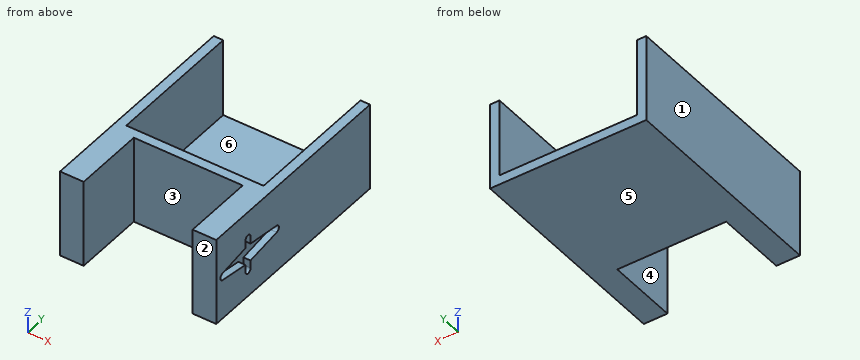
```python
from build123d import *

# Parameters (mm, degrees)
SKETCH_W        = 66
SKETCH_H        = 66
PAD_DEPTH       = 37
SKETCH001_W     = 58
SKETCH001_H     = 58
POCKET_DEPTH    = 33
SKETCH002_W     = 10
SKETCH002_H     = 37
PAD001_DEPTH    = 30
SKETCH003_W     = 66
SKETCH003_H     = 37
POCKET001_DEPTH = 4
POCKET002_DEPTH = 3


with BuildPart() as part:
    # Sketch → Pad (new body)
    with BuildSketch(Plane.XY):
        Rectangle(SKETCH_W, SKETCH_H)
    extrude(amount=PAD_DEPTH)

    # Sketch001 → Pocket (cut)
    with BuildSketch(Plane.XY.offset(37)):
        Rectangle(SKETCH001_W, SKETCH001_H)
    extrude(amount=-POCKET_DEPTH, mode=Mode.SUBTRACT)

    # Sketch002 → Pad001 (new body)
    with BuildSketch(Plane.XZ.offset(33)):
        with Locations((-28, 18.5)):
            Rectangle(SKETCH002_W, SKETCH002_H)
        with Locations((28, 18.5)):
            Rectangle(SKETCH002_W, SKETCH002_H)
    extrude(amount=PAD001_DEPTH)

    # Sketch003 → Pocket001 (cut)
    with BuildSketch(Plane(origin=(0, 33, 0), x_dir=(-1, 0, 0), z_dir=(0, 1, 0))):
        with Locations((0, 18.5)):
            Rectangle(SKETCH003_W, SKETCH003_H)
    extrude(amount=-POCKET001_DEPTH, mode=Mode.SUBTRACT)

    # Sketch005 → Pocket002 (cut)
    with BuildSketch(Plane.YZ.offset(33)):
        with BuildLine():
            Line((-45.5, 22.09772), (-45.5, 25.389621))
            ThreePointArc((-42.5, 25.389621), (-44, 26.889621), (-45.5, 25.389621))
            Line((-42.5, 25.389621), (-42.5, 22.09772))
            Line((-42.5, 22.09772), (-26.789852, 19.874827))
            ThreePointArc((-26.789852, 16.904415), (-25.5, 18.389621), (-26.789852, 19.874827))
            Line((-26.789852, 16.904415), (-42.5, 14.681522))
            Line((-42.5, 14.681522), (-42.5, 11.389621))
            ThreePointArc((-45.5, 11.389621), (-44, 9.889621), (-42.5, 11.389621))
            Line((-45.5, 11.389621), (-45.5, 14.681522))
            Line((-45.5, 14.681522), (-59.240035, 16.908951))
            ThreePointArc((-59.240035, 19.870291), (-60.5, 18.389621), (-59.240035, 16.908951))
            Line((-59.240035, 19.870291), (-45.5, 22.09772))
        make_face()
    extrude(amount=-POCKET002_DEPTH, mode=Mode.SUBTRACT)


solid = part.part
```
Input: part model. Units: mm. Frame: model coordinates. Face numbers are marked on the shaded views. A direction names the side the tool comes from. Coordinates: 2 decimals unless noted, no trailing zeros. Loops run counter-clockwise (first coordinate to the right, second up) from the corner with the lowest first, then second, coordinate; pieces in that order, holes last. Notation, with made-up numbers: M 73,53 L 82,53 A13 ccw 82,70 Z; hole C 85,-28 d9. An arc over 180 degrees is marked long. Use a Markdown table: item, result. Add a question column.
1) Section D-D, the plane x = -20. Return the cut outline in (y, z).
2) Section B-B, the plane z = 35.5. Return the cut outline in (x, y).
3) Pin query (flat end, axial travel): P1, Ø8, axis at x = 15, y = -17.5, coming from the +Z side; P2, Ø10, axis at x = 8, z = 20, coming from the +Y side; P3, Ø2, axis at x = 11, z = 21.5, coming from the -Y side. Return the tip coordinate at first contact, or that it passes through.
4) Section A-A, the plane y = -44. Return the cut outline in (x, z).
5) Draft query along X for the marked faces 1, 2 and 3. Return one class per face: +X half, -X half, draft (parallel to the pull), parting line (faces both ways), or undercut.
6) Section C-C, the plane y = -6. Return the cut outline in (x, z), plus the area to 3 significant figures.
7) Set-up query: the marked faces 4, 5 and 6. Return all of +Z, -Z, +X, -X, +Y, -Y with unobstructed straight access to the full face (end or side cutting, diameter ignored); none if empty.
8) Line query: L1, parallel to X at y = -16.5, z = 17; L2, parallel to X at y = -57, z = 26; L3, parallel to Y at x = -11.5, z = 27. Output: solid intervals per line, ascending. Write a range as from..to.
Answer below:
| question | item | result |
|---|---|---|
| 1 | outline | M -33,0 L 29,0 L 29,4 L -29,4 L -29,37 L -33,37 Z |
| 2 | outline | M -33,-63 L -23,-63 L -23,-33 L 23,-33 L 23,-63 L 33,-63 L 33,29 L 29,29 L 29,-29 L -29,-29 L -29,29 L -33,29 Z |
| 3 | P1 | z = 4 |
| 3 | P2 | y = -29 |
| 3 | P3 | y = -33 |
| 4 | outline | M -33,0 L -23,0 L -23,37 L -33,37 Z; M 23,0 L 33,0 L 33,9.89 L 30,9.89 L 30,26.89 L 33,26.89 L 33,37 L 23,37 Z |
| 5 | face 1 | -X half |
| 5 | face 2 | draft |
| 5 | face 3 | undercut |
| 6 | outline | M -33,0 L 33,0 L 33,37 L 29,37 L 29,4 L -29,4 L -29,37 L -33,37 Z |
| 6 | area | 528 mm2 |
| 7 | face 4 | +Z, -Z, -Y |
| 7 | face 5 | -Z, +X, -X, +Y, -Y |
| 7 | face 6 | +Z, +Y |
| 8 | L1 | -33..-29, 29..33 |
| 8 | L2 | -33..-23, 23..33 |
| 8 | L3 | -33..-29 |
